```python
from build123d import *

# Parameters (mm, degrees)
F0_W     = 152.4
F0_H     = 114.3
F1_DEPTH = 152.4
F2_W     = 114.3
F2_H     = 114.3
F3_DEPTH = 114.3
F4_W     = 38.1
F4_H     = 25.4
F5_DEPTH = 31.75
F6_W     = 31.75
F6_H     = 25.4
F7_DEPTH = 38.101
F8_W     = 50.8
F8_H     = 26.0741613155
F9_DEPTH = 38.101


with BuildPart() as f1:
    # F0 (on Front) → F1 (new body)
    with BuildSketch(Plane.XZ):
        Rectangle(F0_W, F0_H)
    extrude(amount=F1_DEPTH)

    # F2 (on face) → F3 (cut)
    with BuildSketch(Plane.XZ.offset(152.4)):
        with Locations((19.05, 0)):
            Rectangle(F2_W, F2_H)
    extrude(amount=-F3_DEPTH, mode=Mode.SUBTRACT)

    # F4 (on face) → F5 (cut)
    with BuildSketch(Plane.XZ.offset(152.4)):
        with Locations((-57.15, 44.45)):
            Rectangle(F4_W, F4_H)
    extrude(amount=-F5_DEPTH, mode=Mode.SUBTRACT)

    # F6 (on face) → F7 (cut, through all)
    with BuildSketch(Plane.YZ.offset(-38.1)):
        with Locations((-53.975, 44.45)):
            Rectangle(F6_W, F6_H)
    extrude(amount=-F7_DEPTH, mode=Mode.SUBTRACT)

    # F8 (on face) → F9 (cut, through all)
    with BuildSketch(Plane.XZ.offset(38.1)):
        with Locations((0, 44.1129193423)):
            Rectangle(F8_W, F8_H)
    extrude(amount=-F9_DEPTH, mode=Mode.SUBTRACT)


solid = f1.part
```
For this review, take the finished solid that the model builds, in its own axes (mm). A direction names the side the tool comes from. Give positions to 0.01 mm unless a question says otherwise; leave off trailing zeros. Write each loop counter-clockwise with the first axis right and the second up, starting at its lowest first coordinate (ties: lowest second). Pieces come first, ordered by that corner, then holes. Notation, with made-up numbers: M -21.75,-7 L -11.75,-7 A30 cw -11.75,26 Z; hole C 34.5,69.25 d1. An arc over 180 degrees is marked long. Answer as CSV lines item,"result".
1. For faces 5 (the flat face through (-57, -137, 31.75)), 6 (the flat face through (-57, -54, 31.75)), 7 (the flat face through (-38.1, -96, -1)), 8 (the flat face through (25.4, -19, 44)), list the 3-axis set-ups (+Z, -Z, +X, -X, +Y, -Y) from which the entire face can be reached by the end or side of a thin tool; tool diameter is ignored.
Findings:
face 5,"+Z, +X, -X, -Y"
face 6,"+Z, +X, -X"
face 7,"+Z, -Z, +X, -Y"
face 8,"+Z, +Y, -Y"
2. Draft analysis for pull direction X (two halves, no side actions). For faces 1 (the flat face through (76.2, -19, -1)), 2 (the flat face through (-25.4, -19, 44)), 3 (the flat face through (-1, 0, 1)), 4 (the flat face through (0, -19, 31.076)), state which applies: +X half, -X half, draft (parallel to the pull), parting line (faces both ways), or undercut.
Findings:
face 1,"+X half"
face 2,"undercut"
face 3,"draft"
face 4,"undercut"
3. Consider section C-C, the plane x = 32. Write out the cut boundary in (y, z), then the cut area to 3 significant figures.
Findings:
outline,"M -38.1,-57.15 L 0,-57.15 L 0,57.15 L -38.1,57.15 Z"
area,"4,350 mm2"
4. Consider section D-D, the plane z = -31. Write out the cut boundary in (x, y).
Findings:
outline,"M -76.2,-152.4 L -38.1,-152.4 L -38.1,-38.1 L 76.2,-38.1 L 76.2,0 L -76.2,0 Z"
5. For pin 1 (16 mm diameter, centred on x = -50, y = -132.5, fed in from +Z); pin 2 (1 mm diameter, centred on y = -106.5, z = 29.5, fed in from +X); pin 3 (11.5 mm diameter, centred on x = -11.5, y = -19, fed in from +Z), all flat-tipped, find the tip position at first contact; note any pin that passes through.
Findings:
pin 1,"stops at z = 31.75"
pin 2,"stops at x = -38.1"
pin 3,"stops at z = 31.08"
6. Wall thickness on line 1 (X direction, y = -68, z = -23); line 2 (Z direction, x = -50, y = -63); line 3 (Y direction, x = 61, z = -20): over which ranges is each line inside the solid? List them lowest first.
Findings:
line 1,"x = -76.2 to -38.1"
line 2,"z = -57.15 to 31.75"
line 3,"y = -38.1 to 0"
7. Consider section A-A, the plane z = 47.5. Write out the cut boundary in (x, y), then the cut area to 3 significant figures.
Findings:
outline,"M -76.2,-120.65 L -38.1,-120.65 L -38.1,-69.85 L -76.2,-69.85 Z; M -76.2,-38.1 L -25.4,-38.1 L -25.4,0 L -76.2,0 Z; M 25.4,-38.1 L 76.2,-38.1 L 76.2,0 L 25.4,0 Z"
area,"5,810 mm2"
8. Consider section B-B, the plane y = -18. Write out the cut boundary in (x, z).
Findings:
outline,"M -76.2,-57.15 L 76.2,-57.15 L 76.2,57.15 L 25.4,57.15 L 25.4,31.08 L -25.4,31.08 L -25.4,57.15 L -76.2,57.15 Z"
